Verification items for the finished model (mm, model axes). Face numbers are marked on the shaded views. A direction names the side the tool comes from. Round coordinates to 2 decimals unless told otherwise and drop trailing zeros. Loops run counter-clockwise (first coordinate to the right, second up) from the corner with the lowest first, then second, coordinate; pieces in that order, holes last. Notation, with made-up numbers: (20.5, 46) -> (39.5, 46) arc R20 cw to (39.5, 58) -> close; hole circle Ø7 at (30.25, 34). An arc over 180 degrees is marked (long way). Write item = value, one per line.
```python
from build123d import *

# Parameters (mm, degrees)
SZKIC1_R                    = 4.5
SZKIC1_R_2                  = 0.5
DODANIE_WYCI_GNI_CIE1_DEPTH = 2
SZKIC2_W                    = 1.1
SZKIC2_H                    = 1.1
WYTNIJ_WYCI_GNI_CIE1_DEPTH  = 1


with BuildPart() as part:
    # Szkic1 → Dodanie-wyciągnięcie1 (new body)
    with BuildSketch(Plane.XY):
        Circle(SZKIC1_R)
        Circle(SZKIC1_R_2, mode=Mode.SUBTRACT)
    extrude(amount=DODANIE_WYCI_GNI_CIE1_DEPTH)

    # Szkic2 → Wytnij-wyciągnięcie1 (cut)
    with BuildSketch(Plane.XY.offset(2)):
        Polygon((1.315931733, 4.00018108), (0.83865962, 3.009115325), (1.829725375, 2.531843212), (2.306997488, 3.522908967), align=None)
        with Locations((0, 3.625)):
            Rectangle(SZKIC2_W, SZKIC2_H)
        Polygon((2.921227048, 3.033077238), (2.061212418, 2.347238456), (2.7470512, 1.487223825), (3.60706583, 2.173062607), align=None)
        Polygon((3.94793752, 1.465235251), (2.875516816, 1.220462224), (3.120289844, 0.14804152), (4.192710547, 0.392814548), align=None)
        Polygon((4.192710547, -0.392814548), (3.120289844, -0.14804152), (2.875516816, -1.220462224), (3.94793752, -1.465235251), align=None)
        Polygon((3.60706583, -2.173062607), (2.7470512, -1.487223825), (2.061212418, -2.347238456), (2.921227048, -3.033077238), align=None)
        Polygon((2.306997488, -3.522908967), (1.829725375, -2.531843212), (0.83865962, -3.009115325), (1.315931733, -4.00018108), align=None)
        with Locations((0, -3.625)):
            Rectangle(SZKIC2_W, SZKIC2_H)
        Polygon((-1.315931733, -4.00018108), (-0.83865962, -3.009115325), (-1.829725375, -2.531843212), (-2.306997488, -3.522908967), align=None)
        Polygon((-2.921227048, -3.033077238), (-2.061212418, -2.347238456), (-2.7470512, -1.487223825), (-3.60706583, -2.173062607), align=None)
        Polygon((-3.94793752, -1.465235251), (-2.875516816, -1.220462224), (-3.120289844, -0.14804152), (-4.192710547, -0.392814548), align=None)
        Polygon((-4.192710547, 0.392814548), (-3.120289844, 0.14804152), (-2.875516816, 1.220462224), (-3.94793752, 1.465235251), align=None)
        Polygon((-3.60706583, 2.173062607), (-2.7470512, 1.487223825), (-2.061212418, 2.347238456), (-2.921227048, 3.033077238), align=None)
        Polygon((-2.306997488, 3.522908967), (-1.829725375, 2.531843212), (-0.83865962, 3.009115325), (-1.315931733, 4.00018108), align=None)
    extrude(amount=-WYTNIJ_WYCI_GNI_CIE1_DEPTH, mode=Mode.SUBTRACT)


solid = part.part
```
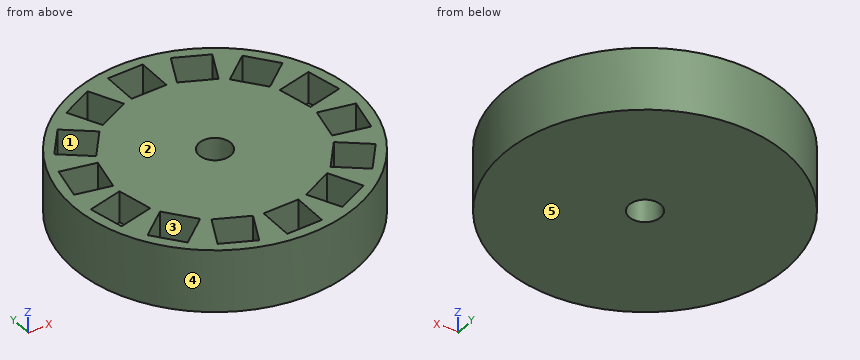
(1) Material ranges on probe 1 along Y at (x, z) = (0, 1.4) (3 decimals); probe 2 along Y at (x, z) = (0, 0.7); probe 3 along X at (y, z) = (3.75, 1.7), recorded low to high. Write a range as from..to.
Filled sheet:
probe_1 = -4.5..-4.175, -3.075..-0.5, 0.5..3.075, 4.175..4.5
probe_2 = -4.5..-0.5, 0.5..4.5
probe_3 = -2.49..-1.84, -1.2..-0.55, 0.55..1.2, 1.84..2.49
(2) Set-up check for the marked faces 1 and 2: record each of +Z, -Z, +X, -X, +Y, -Y from which the full face is reachable in a straight line by a thin tool's end or side.
Filled sheet:
face_1 = +Z
face_2 = +Z, +X, -X, +Y, -Y
(3) Sectioned sample at C-C, the plane z = 0.25. Record the cut outline in (x, y).
Filled sheet:
outline = circle Ø9 at (0, 0); hole circle Ø1 at (0, 0)
(4) Sectioned sample at A-A, the plane y = 0. Record the cut outline in (x, z).
Filled sheet:
outline = (-4.5, 0) -> (-0.5, 0) -> (-0.5, 2) -> (-4.5, 2) -> close; (0.5, 0) -> (4.5, 0) -> (4.5, 2) -> (0.5, 2) -> close
(5) Sectioned sample at D-D, the plane x = -3.75. Record the cut outline in (y, z).
Filled sheet:
outline = (-2.49, 0) -> (2.49, 0) -> (2.49, 2) -> (1.42, 2) -> (1.42, 1) -> (0.29, 1) -> (0.29, 2) -> (-0.29, 2) -> (-0.29, 1) -> (-1.42, 1) -> (-1.42, 2) -> (-2.49, 2) -> close
(6) Draft check along X on the marked faces 3, 4 and 5. Enter one of: released by +X, released by -X, zero draft, split by the parting line, or undercut.
Filled sheet:
face_3 = undercut
face_4 = split by the parting line
face_5 = zero draft
(7) Sectioned sample at B-B, the plane x = 0. Record the cut outline in (y, z) (3 decimals).
Filled sheet:
outline = (-4.5, 0) -> (-0.5, 0) -> (-0.5, 2) -> (-3.075, 2) -> (-3.075, 1) -> (-4.175, 1) -> (-4.175, 2) -> (-4.5, 2) -> close; (0.5, 0) -> (4.5, 0) -> (4.5, 2) -> (4.175, 2) -> (4.175, 1) -> (3.075, 1) -> (3.075, 2) -> (0.5, 2) -> close
(8) Go/stop test with flat-tipped pins: pin 1 Ø0.5 at (y, z) = (3.5, 1.5) entering from +X; pin 2 Ø1.1 at (y, z) = (3.5, 1.5) entering from -X. Record where each tip stops, or that it passes through.
Filled sheet:
pin_1 = 3.11
pin_2 = -3.4
